from build123d import *

# Parameters (mm, degrees)
SKETCH032_R             = 1.8
PAD023_DEPTH            = 5
PAD024_DEPTH            = 80
SKETCH031_R             = 5.2
PAD022_DEPTH            = 80
SKETCH029_R             = 1.5
POCKET006_DEPTH         = 15
BODY004_PLACEMENT_ANGLE = 45


with BuildPart() as part:
    # Sketch032 → Pad023 (new body)
    with BuildSketch(Plane.XY):
        with BuildLine():
            ThreePointArc((59.887401, -16.046781), (62, 0), (59.887401, 16.046781))
            ThreePointArc((59.887401, 16.046781), (51.314187, 20.996528), (46.36444, 12.423314))
            ThreePointArc((43.66723, 6.1557), (46.103592, 8.821401), (46.36444, 12.423314))
            ThreePointArc((43.66723, 6.1557), (40, 0), (43.66723, -6.1557))
            ThreePointArc((46.36444, -12.423314), (46.103592, -8.821401), (43.66723, -6.1557))
            ThreePointArc((46.36444, -12.423314), (51.314187, -20.996528), (59.887401, -16.046781))
        make_face()
        with Locations((47, 0)):
            Circle(SKETCH032_R, mode=Mode.SUBTRACT)
        with Locations((55, 0)):
            Circle(SKETCH032_R, mode=Mode.SUBTRACT)
    extrude(amount=-PAD023_DEPTH)

    # Sketch033 → Pad024 (join)
    with BuildSketch(Plane.XY):
        with BuildLine():
            ThreePointArc((59.887401, -16.046781), (62, 0), (59.887401, 16.046781))
            ThreePointArc((59.887401, 16.046781), (51.314187, 20.996528), (46.36444, 12.423314))
            ThreePointArc((43.66723, 6.1557), (46.103592, 8.821401), (46.36444, 12.423314))
            ThreePointArc((43.66723, 6.1557), (40, 0), (43.66723, -6.1557))
            ThreePointArc((46.36444, -12.423314), (46.103592, -8.821401), (43.66723, -6.1557))
            ThreePointArc((46.36444, -12.423314), (51.314187, -20.996528), (59.887401, -16.046781))
        make_face()
        with BuildLine():
            ThreePointArc((57.95555, 15.529143), (51.831825, 19.064677), (48.296291, 12.940952))
            ThreePointArc((44.61945, 4.396929), (47.940703, 8.030817), (48.296291, 12.940952))
            ThreePointArc((44.61945, 4.396929), (42, 0), (44.61945, -4.396929))
            ThreePointArc((48.296291, -12.940952), (47.940703, -8.030817), (44.61945, -4.396929))
            ThreePointArc((48.296291, -12.940952), (51.831825, -19.064677), (57.95555, -15.529143))
            ThreePointArc((57.95555, -15.529143), (60, 0), (57.95555, 15.529143))
        make_face(mode=Mode.SUBTRACT)
    extrude(amount=-PAD024_DEPTH)

    # Sketch031 → Pad022 (join)
    with BuildSketch(Plane.XY):
        with Locations((53.12592, 14.235047)):
            Circle(SKETCH031_R)
        with Locations((53.12592, -14.235047)):
            Circle(SKETCH031_R)
    extrude(amount=-PAD022_DEPTH)

    # Sketch029 → Pocket006 (cut)
    with BuildSketch(Plane.XY.offset(-80)):
        with Locations((53.12592, 14.235047)):
            Circle(SKETCH029_R)
        with Locations((53.12592, -14.235047)):
            Circle(SKETCH029_R)
    extrude(amount=POCKET006_DEPTH, mode=Mode.SUBTRACT)


with BuildPart() as part_1:
    # Body004 placement: moved
    add(part.part.moved(Location((0, 0, -55))).rotate(Axis((0, 0, -55), (0, 0, 1)), BODY004_PLACEMENT_ANGLE))


solid = part_1.part
The listing builds one solid part. Answer for the finished solid, in the listing's coordinates (mm). A direction names the side the tool comes from. Give positions to 0.01 mm unless a question says otherwise; leave off trailing zeros. Order: outer loops, then holes, each group sorted by start corner. A loop starts at its lowest first (then second) coordinate and runs counter-clockwise, first axis right, second up. Notation, with made-up numbers: (18, 57) - (72, 57) arc R28 ccw to (72, 89) - close; hole circle Ø5 at (61.25, 49). An arc over 180 degrees is marked (long way). Answer as CSV lines item,"result".
Q1. Determine the mould class of faces 1 (the face through (38.89, 26.34, -94.44)), 2 (the face through (44, 43.68, -94.44)), 3 (the face through (37, 38, -60)) for opening direction Y: pulls with the +Y half, pulls with the -Y half, needs draft (parallel to the pull), parting line crosses it, or undercut.
Answer key:
face 1,"pulls with the -Y half"
face 2,"pulls with the +Y half"
face 3,"undercut"
Q2. Each of these flat-tipped pins is pushed along its axis until it touches: pin 1 Ø1.5 at (y, z) = (50.5, -97.5) entering from +X; pin 2 Ø12 at (x, z) = (26, -69.5) entering from -Y; pin 3 Ø0.9 at (x, y) = (27, 47) entering from -Z; pin 4 Ø1 at (x, y) = (43, 48) entering from +Z. Where does it stop, or does it pass through?
Answer key:
pin 1,"stops at x = 37"
pin 2,"stops at y = 26.34"
pin 3,"stops at z = -120"
pin 4,"passes through"
Q3. A cutting plane is placed at A-A, the plane y = 38. Determine the outline of the cut face in (x, z), and give its area (3 significant figures).
Answer key:
outline,"(26.62, -135) - (28.66, -135) - (28.66, -60) - (37.33, -60) - (37.33, -55) - (26.62, -55) - close; (40.45, -60) - (46.43, -60) - (46.43, -135) - (48.99, -135) - (48.99, -55) - (40.45, -55) - close"
area,"441 mm^2"
Q4. Straight lines are drawn through the part: L1, parallel to Y at x = 27.5, z = -128.25; L2, parallel to X at y = 27, z = -130; L3, parallel to X at y = 29, z = -76. For each, find the intervals that lie inside material, in ascending order.
Answer key:
L1,"y = 29.22 to 40.95, 42.43 to 46.13, 49.13 to 54.63"
L2,"x = 30.05 to 41.62, 42.46 to 46.22, 49.05 to 54.61"
L3,"x = 27.66 to 30.57, 42.65 to 54.47"
Q5. Which of the six approach directions +Z, -Z, +X, -X, +Y, -Y give full straight-line access (tool end or side, diameter ignored) to faces 4 (the face through (48.324, 28.83, -127.605)), 5 (the face through (43, 43, -135))?
Answer key:
face 4,"-Z"
face 5,"-Z, +X, -X, +Y, -Y"
Q6. A cutting plane is placed at D-D, the plane x = 45. Determine the outline of the cut face in (y, z).
Answer key:
outline,"(21.01, -135) - (31.99, -135) - (31.99, -60) - (39.69, -60) - (39.69, -135) - (42.65, -135) - (42.65, -55) - (21.01, -55) - close"
